Input: part model. Units: mm. Frame: model coordinates. A direction names the side the tool comes from. Coordinates: 2 decimals unless noted, no trailing zeros. Write each loop counter-clockwise with the first axis right and the second up, starting at its lowest first coordinate (ties: lowest second). Pieces come first, ordered by that corner, then holes. Notation, with made-up numbers: (-23.5, -11.5) - (-10.5, -11.5) arc R13 cw to (-10.5, 9.5) - close; hole circle Ø2 at (41, 29.5). An arc over 180 degrees is marked (long way). One line per question, with ' | ' between items. Start each with the question number.
1) Section query B-B on z = 25.4. Give the number of separate pieces and of enclosed holes in the cut face, and give its area (3 significant figures).
2) Section query D-D on y = 7.5. Return loops of the section in (x, z).
3) Line query: line 1 (Y direction, x = 17, z = 114); line 2 (Y direction, x = 11, z = 99.5); line 3 (Z direction, x = 14.25, y = 0). Output: solid intervals per line, ascending.
4) Section query C-C on y = 0. Return loops of the section in (x, z).
5) First-contact query: P1, Ø10, axis at y = -2, z = 99.5, coming from the -X side; P2, Ø1.9, axis at x = 2.86, z = 25.4, coming from the -Y side. Flat tips, straight axial feed; report the tip coordinate or a pass-through.
6) Reachability of faces 4 (the flat face through (0, 9.842, 69)), 5 (the flat face through (14, 0, 0)) from +Z, -Z, +X, -X, +Y, -Y: full face, straight path, thin tool, end or side. Return the list, or none.
7) Draft query along X for faces 1 (the cylindrical face through (2.651, 12.973, 26.974)), 2 (the flat face through (-12.7, 13, 69)), 3 (the flat face through (14, 0, 139.7)). Return one class per face: released by +X, released by -X, zero draft, split by the parting line, or undercut.
8) Section query A-A on x = -7. Return loops of the section in (y, z), and give its area (3 significant figures).
```python
from build123d import *

# Parameters (mm, degrees)
F1_DEPTH = 139.7
F2_R     = 1.5875
F3_DEPTH = 31.751
F4_R     = 1.5875
F5_DEPTH = 32.386


with BuildPart() as f1:
    # F0 (on Top) → F1 (new body)
    with BuildSketch(Plane.XY):
        Polygon((12.7, -9.8425), (-12.7, -9.8425), (-12.7, -16.1925), (19.05, -16.1925), (19.05, 16.1925), (-12.7, 16.1925), (-12.7, 9.8425), (12.7, 9.8425), align=None)
    extrude(amount=F1_DEPTH)

    # F2 (on face) → F3 (cut, through all)
    with BuildSketch(Plane.YZ.offset(19.05)):
        with Locations((0, 114.3)):
            Circle(F2_R)
        with Locations((0, 25.4)):
            Circle(F2_R)
    extrude(amount=-F3_DEPTH, mode=Mode.SUBTRACT)

    # F4 (on face) → F5 (cut, through all)
    with BuildSketch(Plane.XZ.offset(16.1925)):
        with Locations((2.8575, 114.3)):
            Circle(F4_R)
        with Locations((2.8575, 25.4)):
            Circle(F4_R)
    extrude(amount=-F5_DEPTH, mode=Mode.SUBTRACT)


solid = f1.part
```
Answer key:
1) separate pieces: 4 | enclosed holes: 0 | area: 468 mm²
2) outline: (12.7, 0) - (19.05, 0) - (19.05, 139.7) - (12.7, 139.7) - close
3) line 1: -16.19 to -1.56, 1.56 to 16.19 | line 2: -16.19 to -9.84, 9.84 to 16.19 | line 3: 0 to 23.81, 26.99 to 112.71, 115.89 to 139.7
4) outline: (12.7, 0) - (19.05, 0) - (19.05, 23.81) - (12.7, 23.81) - close; (12.7, 26.99) - (19.05, 26.99) - (19.05, 112.71) - (12.7, 112.71) - close; (12.7, 115.89) - (19.05, 115.89) - (19.05, 139.7) - (12.7, 139.7) - close
5) P1: x = 12.7 | P2: through
6) face 4: +Z, -Z, -X | face 5: -Z, +X, -X, +Y, -Y
7) face 1: undercut | face 2: released by -X | face 3: zero draft
8) outline: (-16.19, 0) - (-9.84, 0) - (-9.84, 139.7) - (-16.19, 139.7) - close; (9.84, 0) - (16.19, 0) - (16.19, 139.7) - (9.84, 139.7) - close | area: 1,770 mm²
